Check sheet for the drawn part. Datum: minimum x, y, z corner. Units: mm. Round coordinates to 2 decimals unless told otherwise and drop trailing zeros. Loops run counter-clockwise (first coordinate to the right, second up) from the corner with the lowest first, then second, coordinate; pieces in that order, holes last. Notation, with made-up numbers: (-1.75, -33) -> (19.25, -33) arc R29 cw to (19.25, -1) -> close; hole circle Ø2 at (17, -6). An arc over 180 degrees is marked (long way). Use CSV: the item, a comma, the result in double quotes. Start each with the question number.
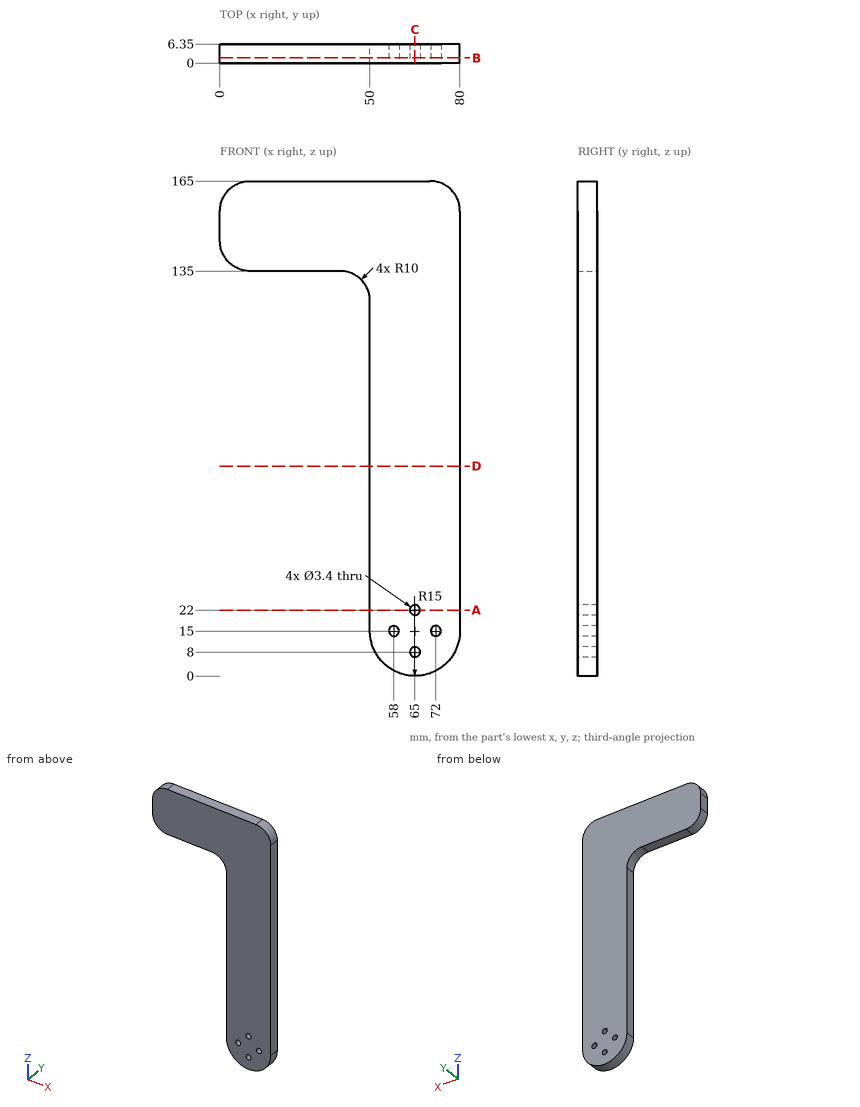
Q1. Thickness scan on L1, parallel to Z at x = 65, y = 3.25; L2, parallel to X at y = 2.75, z = 35.5; L3, parallel to Z at x = 72, y = 3.25. Record the ranges inside material, lowest first. Write a range as from..to.
Q2. Cross-section at A-A (z = 22). Record the boundary of the cut face in (x, y).
Q3. Cross-section at B-B (y = 1.75). Record the boundary of the cut face in (x, z).
Q4. Cross-section at D-D (z = 70). Record the boundary of the cut face in (x, y), and give its area (4 significant figures).
Q5. Cross-section at C-C (x = 65). Record the boundary of the cut face in (y, z).
Q6. Depth check by flat-ended pin: pin 1 Ø4 at (x, z) = (65, 8) entering from +Y. Enter the tip coordinate at first touch or a pass-through.
Answer list:
1,L1,"z = 0..6.3, 9.7..20.3, 23.7..165"
1,L2,"x = 50..80"
1,L3,"z = 1.73..13.3, 16.7..164.8"
2,outline,"(50, 0) -> (63.3, 0) -> (63.3, 6.35) -> (50, 6.35) -> close; (66.7, 0) -> (80, 0) -> (80, 6.35) -> (66.7, 6.35) -> close"
3,outline,"(0, 145) arc R10 ccw to (10, 135) -> (40, 135) arc R10 cw to (50, 125) -> (50, 15) arc R15 ccw to (80, 15) -> (80, 155) arc R10 ccw to (70, 165) -> (10, 165) arc R10 ccw to (0, 155) -> close; hole circle Ø3.4 at (58, 15); hole circle Ø3.4 at (65, 8); hole circle Ø3.4 at (65, 22); hole circle Ø3.4 at (72, 15)"
4,outline,"(50, 0) -> (80, 0) -> (80, 6.35) -> (50, 6.35) -> close"
4,area,"190.5 mm2"
5,outline,"(0, 0) -> (6.35, 0) -> (6.35, 6.3) -> (0, 6.3) -> close; (0, 9.7) -> (6.35, 9.7) -> (6.35, 20.3) -> (0, 20.3) -> close; (0, 23.7) -> (6.35, 23.7) -> (6.35, 165) -> (0, 165) -> close"
6,pin 1,"stops at y = 6.35"
